Print and shaded views of the part. All mm, measured from the part's lowest x, y and z. Round coordinates to 2 decimals unless told otherwise and drop trailing zeros. Write each loop counter-clockwise with the first axis right and the second up, starting at its lowest first coordinate (ties: lowest second). Pieces come first, ordered by that corner, then holes. Notation, with made-up numbers: M -12,-31.5 L 13,-31.5 A20 cw 13,-24.5 Z; hole C 39,78 d5. An arc over 180 degrees is marked long. Write item = value, one per line.
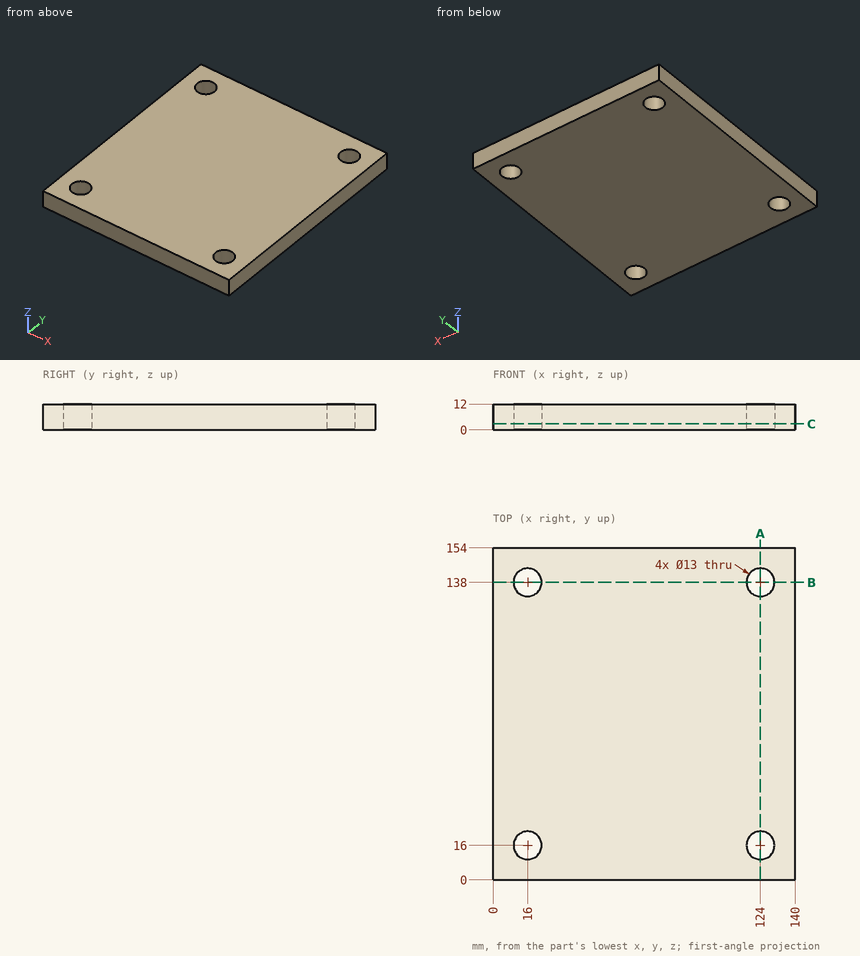
1. Band-saw the part on C-C (z = 2.75). List the corners of the cut face in (x, y), plus the area to 3 significant figures.
Responses:
outline = M 0,0 L 140,0 L 140,154 L 0,154 Z; hole C 16,16 d13; hole C 16,138 d13; hole C 124,16 d13; hole C 124,138 d13
area = 21,000 mm²
2. Probe probe 1 along Y at (x, z) = (124, 3); probe 2 along Y at (x, z) = (119.5, 2.25); probe 3 along X at (y, z) = (139, 7). List the from-to ranges inside material, lowest first.
Responses:
probe_1 = 0 to 9.5, 22.5 to 131.5, 144.5 to 154
probe_2 = 0 to 11.31, 20.69 to 133.31, 142.69 to 154
probe_3 = 0 to 9.58, 22.42 to 117.58, 130.42 to 140
3. Band-saw the part on A-A (x = 124). List the corners of the cut face in (y, z).
Responses:
outline = M 0,0 L 9.5,0 L 9.5,12 L 0,12 Z; M 22.5,0 L 131.5,0 L 131.5,12 L 22.5,12 Z; M 144.5,0 L 154,0 L 154,12 L 144.5,12 Z
4. Band-saw the part on B-B (y = 138). List the corners of the cut face in (x, z).
Responses:
outline = M 0,0 L 9.5,0 L 9.5,12 L 0,12 Z; M 22.5,0 L 117.5,0 L 117.5,12 L 22.5,12 Z; M 130.5,0 L 140,0 L 140,12 L 130.5,12 Z
5. Flat gauge pin, fed straight in: pin 1 (8 mm diameter, centred on x = 16, y = 16, fed in from +Z). Where does the tip first touch, or does it go through?
Responses:
pin_1 = through
